Part model, mm, in its own coordinate system. Give positions to 0.01 mm unless a question says otherwise; leave off trailing zeros. Order: outer loops, then holes, each group sorted by start corner. A loop starts at its lowest first (then second) coordinate and runs counter-clockwise, first axis right, second up. Notation, with made-up numbers: (80, -16.75) - (89, -16.75) arc R22 cw to (89, -3.75) - close; hole circle Ø1 at (79.25, 5.25). An arc over 180 degrees is marked (long way). One line per item, written item: value.
```python
from build123d import *

# Parameters (mm, degrees)
SKETCH1_W           = 530
SKETCH1_H           = 25
BOSS_EXTRUDE3_DEPTH = 2
SKETCH1_5_W         = 27
SKETCH1_5_H         = 19
BOSS_EXTRUDE4_DEPTH = 3
FILLET1_R           = 5
FILLET2_R           = 2.5
FILLET3_R           = 2.5


with BuildPart() as part:
    # Sketch1 → Boss-Extrude3 (new body)
    with BuildSketch(Plane(origin=(0, 0, 0), x_dir=(0, 0, -1), z_dir=(1, 0, 0))):
        Rectangle(SKETCH1_W, SKETCH1_H)
    extrude(amount=-BOSS_EXTRUDE3_DEPTH)

    # Sketch1_5 → Boss-Extrude4 (add)
    with BuildSketch(Plane(origin=(0, 0, 0), x_dir=(0, 0, -1), z_dir=(1, 0, 0))):
        Polygon((-265, 12.5), (-265, -12.5), (0, -12.5), (265, -12.5), (265, 12.5), align=None)
        with Locations((-248.5, 0)):
            Rectangle(SKETCH1_5_W, SKETCH1_5_H, mode=Mode.SUBTRACT)
        Polygon((-232, 9.5), (-101.242640687, 9.5), (-82.242640687, -9.5), (-232, -9.5), align=None, mode=Mode.SUBTRACT)
        Polygon((73.757359313, -9.5), (0, -9.5), (-78, -9.5), (-97, 9.5), (54.757359313, 9.5), align=None, mode=Mode.SUBTRACT)
        with Locations((248.5, 0)):
            Rectangle(SKETCH1_5_W, SKETCH1_5_H, mode=Mode.SUBTRACT)
        Polygon((232, -9.5), (78, -9.5), (59, 9.5), (232, 9.5), align=None, mode=Mode.SUBTRACT)
    extrude(amount=BOSS_EXTRUDE4_DEPTH)

    # Fillet1
    fillet1_edges = [part.edges().sort_by_distance(p)[0] for p in [
        (0.5, 12.5, 265),
        (0.5, 12.5, -265),
        (0.5, -12.5, -265),
        (0.5, -12.5, 265),
    ]]
    fillet(fillet1_edges, radius=FILLET1_R)

    # Fillet2
    fillet2_edges = [part.edges().sort_by_distance(p)[0] for p in [
        (1.5, -9.5, 262),
        (1.5, 9.5, 262),
        (1.5, -9.5, -262),
        (1.5, 9.5, -262),
    ]]
    fillet(fillet2_edges, radius=FILLET2_R)

    # Fillet3
    fillet3_edges = [part.edges().sort_by_distance(p)[0] for p in [
        (1.5, -9.5, 235),
        (1.5, -9.5, -235),
        (1.5, 9.5, -235),
        (1.5, -9.5, -232),
        (1.5, -9.5, -78),
        (1.5, 9.5, -59),
        (1.5, -9.5, -73.757359313),
        (1.5, -9.5, 78),
        (1.5, 9.5, 97),
        (1.5, -9.5, 82.242640687),
        (1.5, -9.5, 232),
        (1.5, 9.5, 232),
        (1.5, 9.5, -232),
        (1.5, 9.5, -54.757359313),
        (1.5, 9.5, 101.242640687),
        (1.5, 9.5, 235),
    ]]
    fillet(fillet3_edges, radius=FILLET3_R)


solid = part.part
```
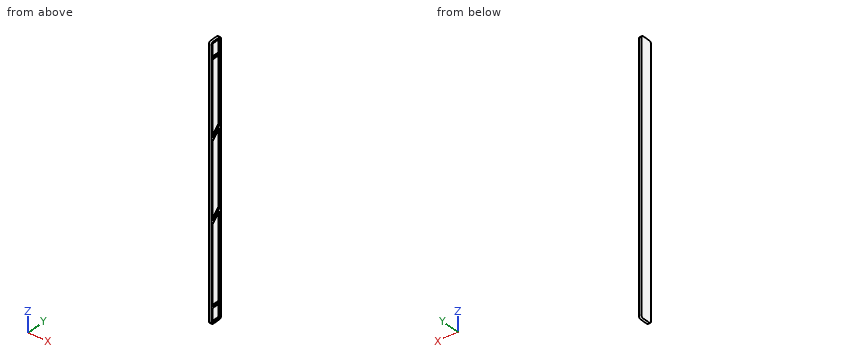
1) Cut at B-B, the plane x = 1.65. Give the number of separate pieces and of enclosed holes in the cut face, then the cut area to 3 significant figures.
Outcome:
separate pieces: 1
enclosed holes: 5
area: 3,600 mm^2
2) Cut at A-A, the plane z = -106. Give the cut face in (x, y), then the cut area to 3 significant figures.
Outcome:
outline: (-2, -12.5) - (3, -12.5) - (3, -9.5) - (0, -9.5) - (0, 9.5) - (3, 9.5) - (3, 12.5) - (-2, 12.5) - close
area: 68.0 mm^2
3) Pin check, flat tip, straight feed: pin 1 (2 mm diameter, centred on y = -2.5, z = -92.5, fed in from +X). Stop position of the tip, or through.
Outcome:
pin 1: stops at x = 0
4) Drill centre lines: line 1 along Y through (x, z) = (0.4, -171); line 2 along Z through (x, y) = (2.5, -9); line 3 along Z through (x, y) = (0.6, -4). Where is each one in solid material? Low to high. Write a range as from..to.
Outcome:
line 1: y = -12.5..-9.5, 9.5..12.5
line 2: z = -264.77..-261, -236..-231, -77.54..-69.22, 78.46..86.78, 231..236, 261..264.77
line 3: z = -265..-262, -235..-232, -72.5..-68.26, 83.5..87.74, 232..235, 262..265
